Source: CAD feature listing. Evaluate the final solid. Frame: model axes, mm. A direction names the side the tool comes from. Round coordinates to 2 decimals unless told otherwise and drop trailing zeros. Write each loop counter-clockwise with the first axis right and the second up, starting at its lowest first coordinate (ties: lowest second). Pieces come first, ordered by that corner, then holes.
from build123d import *

# Parameters (mm, degrees)
SKETCH_1_W          = 72
SKETCH_1_H          = 47
EXTRUDE_1_DEPTH     = 15
SKETCH_2_W          = 62.5
SKETCH_2_H          = 41.5
CUT_EXTRUDE_1_DEPTH = 13
SKETCH_3_R          = 1.5
CUT_EXTRUDE_3_DEPTH = 16
SKETCH_4_W          = 76
SKETCH_4_H          = 51
SKETCH_4_W_2        = 72
SKETCH_4_H_2        = 47
EXTRUDE_2_DEPTH     = 8


with BuildPart() as part:
    # ｽｹｯﾁ1 → ﾎﾞｽ - 押し出し1 (new body)
    with BuildSketch(Plane.XY):
        with Locations((2.027327289, 3.897905759)):
            Rectangle(SKETCH_1_W, SKETCH_1_H)
    extrude(amount=EXTRUDE_1_DEPTH)

    # ｽｹｯﾁ2 → ｶｯﾄ - 押し出し1 (cut)
    with BuildSketch(Plane.XY.offset(15)):
        with Locations((2.027327289, 3.897905759)):
            Rectangle(SKETCH_2_W, SKETCH_2_H)
    extrude(amount=-CUT_EXTRUDE_1_DEPTH, mode=Mode.SUBTRACT)

    # ｽｹｯﾁ3 → ｶｯﾄ - 押し出し3 (cut, through all)
    with BuildSketch(Plane.XY.offset(15)):
        with Locations((-31.472672711, 24.897905759)):
            Circle(SKETCH_3_R)
        with Locations((35.527327289, 24.897905759)):
            Circle(SKETCH_3_R)
        with Locations((-31.472672711, -17.102094241)):
            Circle(SKETCH_3_R)
        with Locations((35.527327289, -17.102094241)):
            Circle(SKETCH_3_R)
    extrude(amount=-CUT_EXTRUDE_3_DEPTH, mode=Mode.SUBTRACT)

    # ｽｹｯﾁ4 → ﾎﾞｽ - 押し出し2 (add)
    with BuildSketch(Plane(origin=(0, 0, 0), x_dir=(-1, 0, 0), z_dir=(0, 0, -1))):
        with Locations((-2.027327289, 3.897905759)):
            Rectangle(SKETCH_4_W, SKETCH_4_H)
        with Locations((-2.027327289, 3.897905759)):
            Rectangle(SKETCH_4_W_2, SKETCH_4_H_2, mode=Mode.SUBTRACT)
    extrude(amount=-EXTRUDE_2_DEPTH)


solid = part.part
1) Pull-direction query (X, two-part tool) for faces 1 (the face through (38.027, 4, 11)), 2 (the face through (34.03, 24.96, 7.6)), 3 (the face through (3, 29.398, 4)), 4 (the face through (2, 24.648, 9)); classes: released by +X, released by -X, zero draft, split by the parting line, or undercut.
Taken from the geometry:
face 1: released by +X
face 2: undercut
face 3: zero draft
face 4: undercut
2) Reachability of faces 5 (the face through (-33.973, 4, 11)), 6 (the face through (2, 27.398, 11)), 7 (the face through (2, -16.852, 9)), 8 (the face through (-32.663, -18.015, 7.605)) from +Z, -Z, +X, -X, +Y, -Y: full face, straight path, thin tool, end or side. Return the list, or none.
Taken from the geometry:
face 5: +Z, -X, +Y, -Y
face 6: +Z, +X, -X, +Y
face 7: +Z
face 8: +Z, -Z
3) Contact query for flat-ended pins moving along their axis: P1, Ø3.5, axis at x = -11.5, z = 11.5, coming from the -Y side; P2, Ø2, axis at x = -13, z = 10, coming from the +Y side; P3, Ø3.5, axis at y = 11, z = 11, coming from the -X side. Output: stop coordinate, or through.
Taken from the geometry:
P1: stops at y = -19.6
P2: stops at y = 27.4
P3: stops at x = -33.97
4) Section query B-B on x = -26. Return the cut outline in (y, z).
Taken from the geometry:
outline: (-21.6, 0) - (29.4, 0) - (29.4, 8) - (27.4, 8) - (27.4, 15) - (24.65, 15) - (24.65, 2) - (-16.85, 2) - (-16.85, 15) - (-19.6, 15) - (-19.6, 8) - (-21.6, 8) - close
5) Section query A-A on z = 3.25. Return the cut outline in (x, y).
Taken from the geometry:
outline: (-35.97, -21.6) - (40.03, -21.6) - (40.03, 29.4) - (-35.97, 29.4) - close; hole circle Ø3 at (-31.47, -17.1); hole circle Ø3 at (-31.47, 24.9); hole (-29.22, -16.85) - (33.28, -16.85) - (33.28, 24.65) - (-29.22, 24.65) - close; hole circle Ø3 at (35.53, -17.1); hole circle Ø3 at (35.53, 24.9)
6) Material intervals for line 1 (X direction, y = 25, z = 9); line 2 (X direction, y = 6, z = 4.5); line 3 (Y direction, x = -7, z = 13), sorted ascending.
Taken from the geometry:
line 1: x = -33.97 to -32.97, -29.98 to 34.03, 37.02 to 38.03
line 2: x = -35.97 to -29.22, 33.28 to 40.03
line 3: y = -19.6 to -16.85, 24.65 to 27.4
7) Section query C-C on y = 17. Return the cut outline in (x, z), then the cut area to 4 significant figures.
Taken from the geometry:
outline: (-35.97, 0) - (40.03, 0) - (40.03, 8) - (38.03, 8) - (38.03, 15) - (33.28, 15) - (33.28, 2) - (-29.22, 2) - (-29.22, 15) - (-33.97, 15) - (-33.97, 8) - (-35.97, 8) - close
area: 299.5 mm2
